from build123d import *

# Parameters (mm, degrees)
BOSS_EXTRUDE1_DEPTH     = 3.175
CUT_EXTRUDE1_DEPTH      = 295.659843082
CUT_EXTRUDE1_DEPTH_BACK = 3.175
SKETCH2_R               = 1.524
CUT_EXTRUDE2_DEPTH      = 5.715
SKETCH4_R               = 1.5621
CUT_EXTRUDE3_DEPTH      = 10.16
SKETCH5_W               = 12.7
SKETCH5_H               = 3.175
SKETCH5_W_2             = 25.4
CUT_EXTRUDE4_DEPTH      = 7.62
SKETCH7_R               = 2.0955
CUT_EXTRUDE5_DEPTH      = 7.62


with BuildPart() as part:
    # Sketch1 → Boss-Extrude1 (new body)
    with BuildSketch(Plane(origin=(0, 0, 0), x_dir=(1, 0, 0), z_dir=(0, 1, 0))):
        Polygon((3.175, 209.55), (0, 209.55), (0, 196.85), (3.175, 196.85), (3.175, 184.15), (0, 184.15), (0, 171.45), (3.175, 171.45), (3.175, 63.5), (0, 63.5), (0, 50.8), (3.175, 50.8), (3.175, 38.1), (0, 38.1), (0, 25.4), (3.175, 25.4), (3.175, 12.7), (0, 12.7), (0, 0), (177.8, 0), (177.8, 12.7), (174.625, 12.7), (174.625, 25.4), (177.8, 25.4), (177.8, 38.1), (174.625, 38.1), (174.625, 50.8), (177.8, 50.8), (177.8, 63.5), (174.625, 63.5), (174.625, 171.45), (177.8, 171.45), (177.8, 184.15), (174.625, 184.15), (174.625, 196.85), (177.8, 196.85), (177.8, 209.55), (174.625, 209.55), (174.625, 222.25), (177.8, 222.25), (177.8, 234.95), (0, 234.95), (0, 222.25), (3.175, 222.25), align=None)
    extrude(amount=BOSS_EXTRUDE1_DEPTH)

    # Sketch2 → Cut-Extrude1 (cut, two sides: drawn at the far end of the back side and taken through both)
    with BuildSketch(Plane(origin=(0, 3.175, 0), x_dir=(1, 0, 0), z_dir=(0, 1, 0)).offset(-CUT_EXTRUDE1_DEPTH_BACK)):
        with BuildLine():
            ThreePointArc((30.5816, 186.8424), (29.0576, 185.3184), (30.5816, 183.7944))
            Line((30.5816, 183.7944), (30.5816, 186.8424))
        make_face()
        with BuildLine():
            Line((30.5816, 186.8424), (30.5816, 183.7944))
            ThreePointArc((30.5816, 183.7944), (31.659230735, 184.240769265), (32.1056, 185.3184))
            ThreePointArc((32.1056, 185.3184), (31.659230735, 186.396030735), (30.5816, 186.8424))
        make_face()
        with BuildLine():
            ThreePointArc((30.5816, 51.1556), (29.0576, 49.6316), (30.5816, 48.1076))
            Line((30.5816, 48.1076), (30.5816, 49.6316))
            Line((30.5816, 49.6316), (30.5816, 51.1556))
        make_face()
        with BuildLine():
            Line((30.5816, 49.6316), (30.5816, 48.1076))
            ThreePointArc((30.5816, 48.1076), (31.659230735, 48.553969265), (32.1056, 49.6316))
            ThreePointArc((32.1056, 49.6316), (31.659230735, 50.709230735), (30.5816, 51.1556))
            Line((30.5816, 51.1556), (30.5816, 49.6316))
        make_face()
        with Locations(Location((147.2184, 49.6316, 0), (0, 0, 90))):
            Circle(SKETCH2_R)
        with Locations(Location((147.2184, 185.3184, 0), (0, 0, 90))):
            Circle(SKETCH2_R)
    extrude(amount=CUT_EXTRUDE1_DEPTH + CUT_EXTRUDE1_DEPTH_BACK, mode=Mode.SUBTRACT)

    # Sketch3 → Cut-Extrude2 (cut)
    with BuildSketch(Plane(origin=(0, 3.175, 0), x_dir=(1, 0, 0), z_dir=(0, 1, 0))):
        with BuildLine():
            ThreePointArc((71.4, 222.25), (71.165685425, 222.815685425), (70.6, 223.05))
            Line((70.6, 223.05), (70.6, 222.25))
            Line((70.6, 222.25), (71.4, 222.25))
        make_face()
        with BuildLine():
            Line((70.6, 222.25), (70.6, 223.05))
            ThreePointArc((70.6, 223.05), (69.8, 222.25), (70.6, 221.45))
            Line((70.6, 221.45), (70.6, 222.25))
        make_face()
        with BuildLine():
            ThreePointArc((70.6, 221.45), (71.165685425, 221.684314575), (71.4, 222.25))
            Line((71.4, 222.25), (70.6, 222.25))
            Line((70.6, 222.25), (70.6, 221.45))
        make_face()
        with BuildLine():
            ThreePointArc((108, 222.25), (107.2, 223.05), (106.4, 222.25))
            Line((106.4, 222.25), (107.2, 222.25))
            Line((107.2, 222.25), (107.2, 221.45))
            ThreePointArc((107.2, 221.45), (107.765685425, 221.684314575), (108, 222.25))
        make_face()
        with BuildLine():
            Line((107.2, 222.25), (106.4, 222.25))
            ThreePointArc((106.4, 222.25), (106.634314575, 221.684314575), (107.2, 221.45))
            Line((107.2, 221.45), (107.2, 222.25))
        make_face()
        with BuildLine():
            ThreePointArc((71.4, 185.65), (71.165685425, 186.215685425), (70.6, 186.45))
            Line((70.6, 186.45), (70.6, 185.65))
            Line((70.6, 185.65), (71.4, 185.65))
        make_face()
        with BuildLine():
            Line((70.6, 185.65), (70.6, 186.45))
            ThreePointArc((70.6, 186.45), (70.034314575, 185.084314575), (71.4, 185.65))
            Line((71.4, 185.65), (70.6, 185.65))
        make_face()
        with BuildLine():
            ThreePointArc((108, 185.65), (107.765685425, 186.215685425), (107.2, 186.45))
            Line((107.2, 186.45), (107.2, 185.65))
            Line((107.2, 185.65), (106.4, 185.65))
            ThreePointArc((106.4, 185.65), (107.2, 184.85), (108, 185.65))
        make_face()
        with BuildLine():
            Line((107.2, 185.65), (107.2, 186.45))
            ThreePointArc((107.2, 186.45), (106.634314575, 186.215685425), (106.4, 185.65))
            Line((106.4, 185.65), (107.2, 185.65))
        make_face()
        with BuildLine():
            Line((70.6, 165.8), (70.6, 166.6))
            Line((70.6, 166.6), (71.4, 166.6))
            ThreePointArc((71.4, 166.6), (70.034314575, 167.165685425), (70.6, 165.8))
        make_face()
        with BuildLine():
            Line((71.4, 166.6), (70.6, 166.6))
            Line((70.6, 166.6), (70.6, 165.8))
            ThreePointArc((70.6, 165.8), (71.165685425, 166.034314575), (71.4, 166.6))
        make_face()
        with BuildLine():
            ThreePointArc((108, 166.6), (107.2, 167.4), (106.4, 166.6))
            Line((106.4, 166.6), (107.2, 166.6))
            Line((107.2, 166.6), (107.2, 165.8))
            ThreePointArc((107.2, 165.8), (107.765685425, 166.034314575), (108, 166.6))
        make_face()
        with BuildLine():
            Line((107.2, 166.6), (106.4, 166.6))
            ThreePointArc((106.4, 166.6), (106.634314575, 166.034314575), (107.2, 165.8))
            Line((107.2, 165.8), (107.2, 166.6))
        make_face()
        with BuildLine():
            ThreePointArc((71.4, 130), (71.165685425, 130.565685425), (70.6, 130.8))
            Line((70.6, 130.8), (70.6, 130))
            Line((70.6, 130), (71.4, 130))
        make_face()
        with BuildLine():
            Line((70.6, 130), (70.6, 130.8))
            ThreePointArc((70.6, 130.8), (70.034314575, 129.434314575), (71.4, 130))
            Line((71.4, 130), (70.6, 130))
        make_face()
        with BuildLine():
            ThreePointArc((108, 130), (107.765685425, 130.565685425), (107.2, 130.8))
            Line((107.2, 130.8), (107.2, 130))
            Line((107.2, 130), (106.4, 130))
            ThreePointArc((106.4, 130), (107.2, 129.2), (108, 130))
        make_face()
        with BuildLine():
            Line((107.2, 130), (107.2, 130.8))
            ThreePointArc((107.2, 130.8), (106.634314575, 130.565685425), (106.4, 130))
            Line((106.4, 130), (107.2, 130))
        make_face()
    extrude(amount=-CUT_EXTRUDE2_DEPTH, mode=Mode.SUBTRACT)

    # Sketch4 → Cut-Extrude3 (cut)
    with BuildSketch(Plane(origin=(0, 3.175, 0), x_dir=(1, 0, 0), z_dir=(0, 1, 0))):
        with Locations(Location((64.7319, 20.32, 0), (0, 0, 270))):
            Circle(SKETCH4_R)
        with Locations(Location((113.0681, 20.32, 0), (0, 0, 270))):
            Circle(SKETCH4_R)
        with Locations(Location((64.7319, 102.9462, 0), (0, 0, 270))):
            Circle(SKETCH4_R)
        with Locations(Location((113.0681, 95.4532, 0), (0, 0, 270))):
            Circle(SKETCH4_R)
    extrude(amount=-CUT_EXTRUDE3_DEPTH, mode=Mode.SUBTRACT)

    # Sketch5 → Cut-Extrude4 (cut)
    with BuildSketch(Plane(origin=(0, 3.175, 0), x_dir=(1, 0, 0), z_dir=(0, 1, 0))):
        with Locations((19.05, 1.5875)):
            Rectangle(SKETCH5_W, SKETCH5_H)
        with Locations((44.45, 1.5875)):
            Rectangle(SKETCH5_W, SKETCH5_H)
        with Locations((76.2, 1.5875)):
            Rectangle(SKETCH5_W_2, SKETCH5_H)
        with Locations((101.6, 1.5875)):
            Rectangle(SKETCH5_W_2, SKETCH5_H)
        with Locations((133.35, 1.5875)):
            Rectangle(SKETCH5_W, SKETCH5_H)
        with Locations((158.75, 1.5875)):
            Rectangle(SKETCH5_W, SKETCH5_H)
    cut_extrude4 = extrude(amount=-CUT_EXTRUDE4_DEPTH, mode=Mode.SUBTRACT)

    # Mirror1: Cut-Extrude4 across plane
    add(cut_extrude4.mirror(Plane.XY.offset(-117.475)), mode=Mode.SUBTRACT)

    # Sketch7 → Cut-Extrude5 (cut)
    with BuildSketch(Plane.XZ):
        with Locations(Location((41.8719, -77.2795, 0), (0, 0, 270))):
            Circle(SKETCH7_R)
        with Locations(Location((41.8719, -157.6705, 0), (0, 0, 90))):
            Circle(SKETCH7_R)
    extrude(amount=-CUT_EXTRUDE5_DEPTH, mode=Mode.SUBTRACT)


solid = part.part
CAD build for the part. Positions are in the model's coordinates, mm. Give positions to 0.01 mm unless a question says otherwise; leave off trailing zeros. Order: outer loops, then holes, each group sorted by start corner. A loop starts at its lowest first (then second) coordinate and runs counter-clockwise, first axis right, second up. Notation, with made-up numbers: (29, 2) -> (38, 2) arc R7 ccw to (38, 14) -> close; hole circle Ø9 at (-14, 39.5). An arc over 180 degrees is marked (long way). Return JSON: item names as keys, results as strings.
Q1. Flat gauge pins, fed straight in: pin 1 (3 mm diameter, centred on x = 64.73, z = -20.32, fed in from -Y); pin 2 (1 mm diameter, centred on y = 1, z = -216.5, fed in from -X) (3 decimals); pin 3 (1.6 mm diameter, centred on x = 156, y = 2.5, fed in from -Z) (3 decimals). Where does each tip first touch, or does it go through?
Working result:
{"pin 1": "through", "pin 2": "x = 3.175", "pin 3": "z = -231.775"}
Q2. Saw through at A-A (x = 15.5). Write the cut outline in (y, z) (3 decimals), then the cut area to 3 significant figures.
Working result:
{"outline": "(0, -231.775) -> (3.175, -231.775) -> (3.175, -3.175) -> (0, -3.175) -> close", "area": "726 mm²"}
Q3. Saw through at B-B (z = -41). Write the cut outline in (x, y) (3 decimals).
Working result:
{"outline": "(3.175, 0) -> (174.625, 0) -> (174.625, 3.175) -> (3.175, 3.175) -> close"}
Q4. Saw through at C-C (y = 1.45). Count the separate pieces of the cut face and the enclosed holes in it, then the cut area to 3 significant figures.
Working result:
{"separate pieces": "1", "enclosed holes": "18", "area": "40,000 mm²"}
Q5. Drill centre lines: line 1 (Z direction, x = 70.6, y = 0.8) (3 decimals); line 2 (X direction, y = 1.3, z = -130) (3 decimals); line 3 (X direction, y = 0.75, z = -20.32) (3 decimals). Where is each one in solid material? Low to high.
Working result:
{"line 1": "-231.775 to -223.05, -221.45 to -186.45, -184.85 to -167.4, -165.8 to -130.8, -129.2 to -3.175", "line 2": "3.175 to 69.8, 71.4 to 106.4, 108 to 174.625", "line 3": "3.175 to 63.17, 66.294 to 111.506, 114.63 to 174.625"}
